from build123d import *

# Parameters (mm, degrees)
F1_DEPTH  = 3
F2_R      = 1.075
F3_DEPTH  = 3
F4_R      = 1.075
F5_DEPTH  = 3
F6_W      = 12
F6_H      = 3
F7_DEPTH  = 10
F8_R      = 0.5
F9_DEPTH  = 3
F10_SIZE  = 2
F11_W     = 3
F11_H     = 10
F12_DEPTH = 25
F13_SIZE  = 5


# Not quite as in the source:
# - a feature names something its author has since deleted; it is built from what else it names


with BuildPart() as f1:
    # F0 (on Top) → F1 (new body)
    with BuildSketch(Plane.XY):
        Polygon((30, 56.1203770339), (-30, 56.1203770339), (-50, 41.1203770339), (-50, 16.1203770339), (-42.8093671799, 16.1203770339), (-42.8093671799, -8.8796229661), (-50, -8.8796229661), (-50, -43.8796229661), (50, -43.8796229661), (50, -8.8796229661), (42.8093671799, -8.8796229661), (42.8093671799, 16.1203770339), (50, 16.1203770339), (50, 41.1203770339), align=None)
    extrude(amount=F1_DEPTH)

    # F2 (on face) → F3 (join)
    with BuildSketch(Plane.YZ.offset(42.8093671799)):
        with BuildLine():
            Line((-5.9190149802, 3), (13.1597690481, 3))
            ThreePointArc((13.1597690481, 3), (3.6203770339, 16), (-5.9190149802, 3))
        make_face()
        with Locations((3.6203770339, 6)):
            Circle(F2_R, mode=Mode.SUBTRACT)
    extrude(amount=-F3_DEPTH)

    # F4 (on face) → F5 (join)
    with BuildSketch(Plane(origin=(-42.8093671799, 0, 0), x_dir=(0, -1, 0), z_dir=(-1, 0, 0))):
        with BuildLine():
            Line((-13.1019409746, 3), (5.8611869067, 3))
            ThreePointArc((5.8611869067, 3), (-3.6203770339, 15.9448506656), (-13.1019409746, 3))
        make_face()
        with Locations((-3.6203770339, 6)):
            Circle(F4_R, mode=Mode.SUBTRACT)
    extrude(amount=-F5_DEPTH)

    # F6 (on face) → F7 (join)
    with BuildSketch(Plane.XY.offset(3)):
        with Locations((-24, 54.6203770339)):
            Rectangle(F6_W, F6_H)
        with Locations((24, 54.6203770339)):
            Rectangle(F6_W, F6_H)
    extrude(amount=F7_DEPTH)

    # F8 (on face) → F9 (cut, through all)
    with BuildSketch(Plane(origin=(0, 56.1203770339, 0), x_dir=(-1, 0, 0), z_dir=(0, 1, 0))):
        with Locations((-25.5, 8)):
            Circle(F8_R)
        with Locations((-22.5, 8)):
            Circle(F8_R)
        with Locations((25.5, 8)):
            Circle(F8_R)
        with Locations((22.5, 8)):
            Circle(F8_R)
    extrude(amount=-F9_DEPTH, mode=Mode.SUBTRACT)

    # F10
    f10_edges = [f1.edges().sort_by_distance(p)[0] for p in [
        (18, 54.620377, 13),
        (30, 54.620377, 13),
        (-18, 54.620377, 13),
        (-30, 54.620377, 13),
    ]]
    chamfer(f10_edges, length=F10_SIZE)

    # F11 (on face) → F12 (join)
    with BuildSketch(Plane.XY.offset(3)):
        with Locations((48.5, -38.8796229661)):
            Rectangle(F11_W, F11_H)
        with Locations((-48.5, -38.8796229661)):
            Rectangle(F11_W, F11_H)
    extrude(amount=F12_DEPTH)

    # F13
    f13_edges = [f1.edges().sort_by_distance(p)[0] for p in [
        (-48.5, -33.879623, 28),
        (48.5, -33.879623, 28),
    ]]
    chamfer(f13_edges, length=F13_SIZE)


solid = f1.part
Source: CAD feature listing. Evaluate the final solid. Frame: model axes, mm. A direction names the side the tool comes from. Round coordinates to 2 decimals unless told otherwise and drop trailing zeros. Order: outer loops, then holes, each group sorted by start corner. A loop starts at its lowest first (then second) coordinate and runs counter-clockwise, first axis right, second up. Notation, with made-up numbers: (-17, 29.25) -> (13, 29.25) arc R14 ccw to (13, 33.25) -> close; hole circle Ø5 at (27.25, 87). An arc over 180 degrees is marked (long way). Answer as CSV lines item,"result".
Item 1: Section C-C, the plane x = 8. Return loops of the section in (y, z), plus the area to 3 significant figures.
A:
outline,"(-43.88, 0) -> (56.12, 0) -> (56.12, 3) -> (-43.88, 3) -> close"
area,"300 mm²"
Item 2: Pull-direction query (X, two-part tool) for faces 1 (the face through (-39.809, 4, 8)), 2 (the face through (0, 56.12, 2)), 3 (the face through (47, -39, 15)), 4 (the face through (30, 55, 7)); classes: pulls with the +X half, pulls with the -X half, needs draft (parallel to the pull), parting line crosses it, or undercut.
A:
face 1,"undercut"
face 2,"needs draft"
face 3,"undercut"
face 4,"pulls with the +X half"
Item 3: Section D-D, the plane y = -32. Return loops of the section in (x, z).
A:
outline,"(-50, 0) -> (50, 0) -> (50, 3) -> (-50, 3) -> close"
Item 4: Line query: L1, parallel to Z at x = -25.5, y = 55; L2, parallel to X at y = -36.5, z = 24.75; L3, parallel to Z at x = 17, y = -33.5. Output: solid intervals per line, ascending.
A:
L1,"0 to 7.5, 8.5 to 13"
L2,"-50 to -47, 47 to 50"
L3,"0 to 3"
Item 5: Pin query (flat end, axial travel): pin 1 Ø3.5 at (x, y) = (23.5, 54) entering from +Z; pin 2 Ø2.5 at (y, z) = (54, 6.5) entering from +X; pin 3 Ø10 at (y, z) = (5.5, 9.5) entering from -X. Return the tip coordinate at first contact, or that it passes through.
A:
pin 1,"z = 13"
pin 2,"x = 30"
pin 3,"x = -42.81"
Item 6: Section A-A, the plane z = 17.25. Return loops of the section in (x, y).
A:
outline,"(-50, -43.88) -> (-47, -43.88) -> (-47, -33.88) -> (-50, -33.88) -> close; (47, -43.88) -> (50, -43.88) -> (50, -33.88) -> (47, -33.88) -> close"
Item 7: Section B-B, the plane z = 26.5. Return loops of the section in (x, y), plus the area to 3 significant figures.
A:
outline,"(-50, -43.88) -> (-47, -43.88) -> (-47, -37.38) -> (-50, -37.38) -> close; (47, -43.88) -> (50, -43.88) -> (50, -37.38) -> (47, -37.38) -> close"
area,"39.0 mm²"
Item 8: Reachability of faces 5 (the face through (50, 28, 1)), 6 (the face through (-46, 16.12, 1)), 7 (the face through (46, -8.88, 1)), 8 (the face through (39.809, 3, 8)), 9 (the face through (-0.2, -43.88, 2.5)) from +Z, -Z, +X, -X, +Y, -Y: full face, straight path, thin tool, end or side. Return the list, or none.
A:
face 5,"+Z, -Z, +X, +Y, -Y"
face 6,"+Z, -Z, -X"
face 7,"+Z, -Z, +X"
face 8,"+Z, +Y, -Y"
face 9,"+Z, -Z, +X, -X, -Y"
